Autodesk Inventor part; units mm, degrees
ref_plane "Work Plane2" through (0, 0, -8101) normal (0, 0, 1) x (1, 0, 0)
ref_plane "Work Plane3" through (2600, 0, 0) normal (1, 0, 0) x (0, 1, 0)
ref_plane "Work Plane4" through (2537.8831, 2179.9067, -2717.5683) normal (-0.6423359, -0.7662012, -0.0184479) x (-0.0374831, 0.0554467, -0.9977578)
sketch "Sketch1" plane through (0, 0, 0) normal (0, 0, 1) x (1, 0, 0)
  arc A0 (4796.3585, -1909.6289) -> (3343.4744, 1121.5056) centre (-3903.1767, -4215.7265) ccw
  line L0 (3236.8192, 1046.7661) -> (3343.5051, 1121.464)
  arc A1 (3228.7635, 1285.3391) -> (1546.1726, 3076.3751) centre (-4110.5601, -3923.7232) ccw
  line L1 (3228.7635, 1285.3391) -> (3122.0787, 1210.6419)
  line L2 (1372.9503, 3176.3452) -> (1308.1705, 3064.1503)
  arc A2 (1372.9503, 3176.3452) -> (93.8576, 4024.2684) centre (-4221.2651, -3873.8147) ccw
  line L3 (1481.3729, 2964.1457) -> (1546.1726, 3076.3751)
  arc A3 (4543.4821, -2147.4888) -> (93.8528, 3844.2289) centre (-4256.4671, -4034.5221) ccw
  line L4 (93.8576, 4024.2684) -> (93.8528, 3844.2289)
  line L5 (1308.1705, 3064.1503) -> (1481.3729, 2964.1457)
  line L6 (3122.0787, 1210.6419) -> (3236.8192, 1046.7661)
  arc A4 (4543.4821, -2147.4888) -> (4796.3585, -1909.6289) centre (4134.8595, -1459.7188) ccw
  point P0 (0, 0)
  dimension "d7" = 800
ref_plane "Work Plane2" through (0, 0, -8101) normal (0, 0, 1) x (1, 0, 0)
ref_plane "Work Plane1" through (0, 0, 0) normal (0, 0, 1) x (1, 0, 0)
sketch "Sketch2" plane through (0, 0, -8101) normal (0, 0, 1) x (1, 0, 0)
  arc A0 (1192.0552, 3508.338) -> (93.8528, 4294.485) centre (-5164.5547, -4211.3454) ccw
  arc A1 (3133.8513, 1483.0798) -> (1365.2603, 3408.338) centre (-5051.6105, -4261.3276) ccw
  arc A2 (4543.6426, -2147.8414) -> (93.8528, 4114.0508) centre (-5207.4444, -4365.1147) ccw
  line L0 (1192.0552, 3508.338) -> (1126.9741, 3395.6142)
  line L1 (1365.2603, 3408.338) -> (1300.1792, 3295.6142)
  line L2 (1126.9741, 3395.6142) -> (1300.1792, 3295.6142)
  line L3 (93.8528, 4294.485) -> (93.8528, 4114.0508)
  line L4 (3027.6129, 1408.6909) -> (3133.8513, 1483.0798)
  line L5 (3142.3282, 1244.8605) -> (3248.5665, 1319.2494)
  line L6 (3027.6129, 1408.6909) -> (3142.3282, 1244.8605)
  arc A3 (4803.6655, -1899.2732) -> (3248.5665, 1319.2494) centre (-4832.968, -4570.4704) ccw
  arc A4 (4543.6426, -2147.8414) -> (4803.6655, -1899.2732) centre (4135.0016, -1460.0824) ccw
  point P0 (0, 0)
loft "Loft1" add profiles "Sketch1", "Sketch2"
ref_plane "Work Plane3" through (2600, 0, 0) normal (1, 0, 0) x (0, 1, 0)
sketch "Sketch3" plane through (2600, 0, 0) normal (1, 0, 0) x (0, 1, 0)
  line L0 (3120.8038, -3828.6818) -> (2179.9067, -2717.5683)
  line L1 (2179.9067, -2717.5683) -> (2281.1646, -4539.693)
  line L2 (2281.1646, -4539.693) -> (3120.8038, -3828.6818)
  line L3 (4534.6211, 332.5956) -> (-2270.5383, 332.5956)
  line L4 (-2270.5383, 332.5956) -> (-2270.5383, -8394.1003)
  line L5 (-2270.5383, -8394.1003) -> (4534.6211, -8394.1003)
  line L6 (4534.6211, -8394.1003) -> (4534.6211, 332.5956)
  point P0 (0, 0)
extrude "Extrusion1" cut sketch "Sketch3" along normal through all both and the other way through all
sketch "Sketch5" plane through (2219.0112, 2281.1646, -4539.693) normal (0, -0.9984595, -0.0554857) x (1, 0, 0)
  line L0 (318.8718, 1824.936) -> (250.4195, 0)
  point P0 (-2219.0112, 4659.2715)
ref_plane "Work Plane4" through (2537.8831, 2179.9067, -2717.5683) normal (-0.6423359, -0.7662012, -0.0184479) x (-0.0374831, 0.0554467, -0.9977578)
sketch "Sketch6" plane through (2537.8831, 2179.9067, -2717.5683) normal (-0.6423359, -0.7662012, -0.0184479) x (-0.0374831, 0.0554467, -0.9977578)
  line L0 (-729.0595, -1938.3665) -> (2085.591, -1938.3665)
  line L1 (2085.591, -1938.3665) -> (2085.591, 179.9667)
  line L2 (2085.591, 179.9667) -> (-729.0595, 179.9667)
  line L3 (-729.0595, 179.9667) -> (-729.0595, -1938.3665)
  point P0 (-2737.216, -722.0143)
extrude "Extrusion2" cut sketch "Sketch6" against normal through all
ref_plane "Work Plane5" through (2537.8831, 2179.9067, -2717.5683) normal (-0.9992973, -0.0020798, 0.0374254) x (-0.0374831, 0.0554467, -0.9977578)
sketch "Sketch7" plane through (2537.8831, 2179.9067, -2717.5683) normal (-0.9992973, -0.0020798, 0.0374254) x (-0.0374831, 0.0554467, -0.9977578)
  line L0 (1826.2193, 0) -> (0, 0)
  line L1 (1201.6643, -877.7967) -> (1826.2193, 0)
  line L2 (0, 0) -> (1201.6643, -877.7967)
  point P0 (-2737.216, 2025.7624)
sketch "Sketch8" plane through (2537.8831, 2179.9067, -2717.5683) normal (-0.6423359, -0.7662012, -0.0184479) x (-0.0374831, 0.0554467, -0.9977578)
  line L0 (1826.2193, 0) -> (0, 0)
  line L1 (1201.6643, -1365.6093) -> (1826.2193, 0)
  line L2 (0, 0) -> (1201.6643, -1365.6093)
  point P0 (-2737.216, -722.0143)
loft "Loft2" add profiles "Sketch7" section 1 edges at (2503.6569, 2230.5357, -3628.6306) (1958.4447, 2700.9842, -4184.1874) (1992.6709, 2650.3553, -3273.125)
sketch "Sketch9" plane through (2537.8831, 2179.9067, -2717.5683) normal (0.9992973, 0.0020798, -0.0374254) x (-0.0374831, 0.0554467, -0.9977578)
  line L0 (1201.6643, 877.7967) -> (0, 0)
  line L1 (1826.2193, 0) -> (1201.6643, 877.7967)
  line L2 (1201.6643, 877.7967) -> (1104.7642, 807.0127)
  line L3 (1201.6643, 877.7967) -> (1271.2326, 780.0202)
  line L4 (1271.2326, 780.0202) -> (1352.713, 837.9938)
  line L5 (1104.7642, 807.0127) -> (1045.7775, 887.7628)
  line L6 (1045.7775, 887.7628) -> (1224.4425, 1018.2748)
  line L7 (1352.713, 837.9938) -> (1224.4425, 1018.2748)
  point P0 (-2737.216, -2025.7624)
  dimension "d23" = 120
  dimension "d24" = 120
  dimension "d25" = 100
  dimension "d26" = 100
extrude "Extrusion3" add sketch "Sketch9" against normal blind 1045.9
sketch "Sketch10" plane through (2537.8831, 2179.9067, -2717.5683) normal (0.9992973, 0.0020798, -0.0374254) x (-0.0374831, 0.0554467, -0.9977578)
  spline S0 degree 5 poles (1206.6873, 877.7967) (1235.6092, 837.1011) (1264.8055, 796.0647) (1294.2703, 754.695) (1323.9982, 712.9995) (1384.2838, 628.5301) (1414.847, 585.7495) (1445.6675, 542.6512) (1476.7397, 499.2425) (1539.6833, 411.3906) (1571.5596, 366.9415) (1603.6814, 322.1905) (1636.0432, 277.145) (1701.5649, 186.0221) (1734.7295, 139.9388) (1768.128, 93.5694) (1801.7552, 46.9208) (1835.6058, 0) knots 0 0 0 0 0 0 0.246209 0.246209 0.246209 0.246209 0.495004 0.495004 0.495004 0.495004 0.746236 0.746236 0.746236 0.746236 1 1 1 1 1 1
  line L0 (1104.7642, 807.0127) -> (0, 0)
  line L1 (1826.2193, 0) -> (0, 0)
  line L2 (1835.6058, 0) -> (1826.2193, 0)
  line L3 (1104.7642, 807.0127) -> (1204.9396, 880.1893)
  line L4 (1201.4146, 877.6143) -> (1104.7642, 807.0127)
  line L5 (1206.6873, 877.7967) -> (1204.9396, 880.1893)
  point P0 (-2737.216, -2025.7624)
extrude "Extrusion4" cut sketch "Sketch10" against normal blind 2000
properties part number "panel_block_03" material "Wood (Maple)"
The listing builds one solid part. Answer for the finished solid, in the listing's coordinates (mm). Round coordinates to 2 decimals unless told otherwise and drop trailing zeros. Order: outer loops, then holes, each group sorted by start corner. A loop starts at its lowest first (then second) coordinate and runs counter-clockwise, first axis right, second up. Notation, with made-up numbers: (-20, 24) -> (31, 24) arc R26 cw to (31, 53) -> close; hole circle Ø2 at (84, -9.5). An arc over 180 degrees is marked (long way). Put each result on its own line as item: value.
Q1. Section A-A, the plane y = 3162 is taken. Write down the section's boundary in (x, z).
Results list:
outline: (1444.03, -3923.7) -> (2489.14, -3964.58) -> (2496.88, -3757.74) -> (1451.61, -3721.25) -> close
Q2. Each of these flat-tipped pins is pushed along its axis until it touches: P1, Ø8, axis at x = 2355, z = -3718, coming from the -Y side; P2, Ø8, axis at x = 1637, z = -3746.5, coming from the +Y side; P3, Ø5, axis at x = 1855, z = -3960, coming from the +Y side. Where does it stop, or does it pass through?
Results list:
P1: y = 3104.91
P2: y = 3180.65
P3: y = 3139.82
Q3. Consider line 1 along Z through (x, y) = (1513, 3101.5); line 2 along Z through (x, y) = (2430, 3124); line 3 along X through (y, z) = (3183, -3817). Determine where each line is inside the solid, lowest interval first.
Results list:
line 1: -3974.74 to -3851.9, -3807.39 to -3691.83
line 2: -3992.63 to -3869.78, -3866.89 to -3709.29
line 3: 1447.98 to 2494.62
Q4. Section B-B, the plane z = -3723 is taken. Write down the section's boundary in (x, y), and give its area (3 significant figures).
Results list:
outline: (1451.55, 3163.43) -> (1451.76, 3060.55) -> (2498.29, 3110.54) -> (2498.24, 3133.52) -> close
area: 65,900 mm^2
Q5. Section C-C, the plane z = -3992 is taken. Write down the section's boundary in (x, y), and give its area (3 significant figures).
Results list:
outline: (1719.48, 3090.02) -> (2488.3, 3068.63) -> (2488.18, 3127.64) -> close
area: 22,700 mm^2
